Check sheet for the modelled part. Datum: model origin and axes. Units: mm. Give positions to 0.01 mm unless a question says otherwise; leave off trailing zeros. Order: outer loops, then holes, each group sorted by start corner. A loop starts at its lowest first (then second) coordinate and runs counter-clockwise, first axis right, second up. Notation, with made-up numbers: (45, 36) -> (51, 36) arc R16 ccw to (51, 41) -> close; hole circle Ø3 at (30, 23.5). An arc over 180 degrees is marked (long way). Answer in a Markdown table with one row per item. Add a question column.
(1) Cross-section at D-D (y = -6.5). Record the cut outline in (x, z), then the cut area to 4 significant figures.
(2) Go/stop test with flat-tipped pins: pin 1 (16 mm diameter, centred on x = 0, y = 0, fed in from +Z); pin 2 (10 mm diameter, centred on x = 18, y = -8, fed in from +Z). Record where each tip stops, or that it passes through.
(3) Cross-section at C-C (x = 0). Record the cut outline in (y, z), then the cut area to 3 significant figures.
(4) Cross-section at A-A (z = 4.25). Record the cut outline in (x, y), then the cut area to 3 significant figures.
(5) Cross-section at B-B (y = 0). Record the cut outline in (x, z), then the cut area to 3 significant figures.
(6) Thickness scan on L1, parallel to X at y = 0, z = 2.5; L2, parallel to Y at x = 0, z = 5.75; L3, parallel to X at y = -2.5, z = 1.75. Record the ranges inside material, lowest first. Write a range as [from, to].
```python
from build123d import *

# Parameters (mm, degrees)
F0_W        = 140
F0_H        = 33
F0_R        = 5
F1_DEPTH    = 12
F2_T1_DEPTH = 760.9710283957


# Not quite as in the source:
# - a fillet or chamfer that OpenCascade refuses, or shapes differently, is made with other operations: its cross-section is extruded or revolved along the edge and cut away or added


with BuildPart() as f1:
    # F0 (on Top) → F1 (new body)
    with BuildSketch(Plane.XY):
        with Locations((-0.2143342793, 0.0709771141)):
            Rectangle(F0_W, F0_H)
        Circle(F0_R, mode=Mode.SUBTRACT)
    extrude(amount=F1_DEPTH)

    # F2: chamfer of 6.5 x 140 on 1 edges, made by hand

    # F2_s2 → F2_t1 (cut)
    with BuildSketch(Plane.XZ.offset(-380.556491312)):
        Polygon((69.7856657207, 5.5), (-70.2143342793, 12), (69.7856657207, 12), align=None)
    extrude(amount=F2_T1_DEPTH, mode=Mode.SUBTRACT)


solid = f1.part
```
Answer below:
| question | item | result |
|---|---|---|
| 1 | outline | (-70.21, 0) -> (69.79, 0) -> (69.79, 5.5) -> (-70.21, 12) -> close |
| 1 | area | 1,225 mm² |
| 2 | pin 1 | stops at z = 9.11 |
| 2 | pin 2 | stops at z = 8.14 |
| 3 | outline | (-16.43, 0) -> (-5, 0) -> (-5, 8.74) -> (-16.43, 8.74) -> close; (5, 0) -> (16.57, 0) -> (16.57, 8.74) -> (5, 8.74) -> close |
| 3 | area | 201 mm² |
| 4 | outline | (-70.21, -16.43) -> (69.79, -16.43) -> (69.79, 16.57) -> (-70.21, 16.57) -> close; hole circle Ø10 at (0, 0) |
| 4 | area | 4,540 mm² |
| 5 | outline | (-70.21, 0) -> (-5, 0) -> (-5, 8.97) -> (-70.21, 12) -> close; (5, 0) -> (69.79, 0) -> (69.79, 5.5) -> (5, 8.51) -> close |
| 5 | area | 1,140 mm² |
| 6 | L1 | x = [-70.21, -5], [5, 69.79] |
| 6 | L2 | y = [-16.43, -5], [5, 16.57] |
| 6 | L3 | x = [-70.21, -4.33], [4.33, 69.79] |
